from build123d import *

# Parameters (mm, degrees)
BOSS_EXTRUDE2_DEPTH = 15
SKETCH3_3_R         = 7.5
BOSS_EXTRUDE3_DEPTH = 20


with BuildPart() as part:
    # Sketch3 → Boss-Extrude2 (new body, symmetric)
    with BuildSketch(Plane.XY):
        Polygon((0, 0), (30, -30), (35, -30), (5, 0), align=None)
    extrude(amount=BOSS_EXTRUDE2_DEPTH, both=True)

    # Sketch3<3> → Boss-Extrude3 (add, symmetric)
    with BuildSketch(Plane.XY):
        with Locations((0.5, 6)):
            Circle(SKETCH3_3_R)
    extrude(amount=BOSS_EXTRUDE3_DEPTH, both=True)


solid = part.part
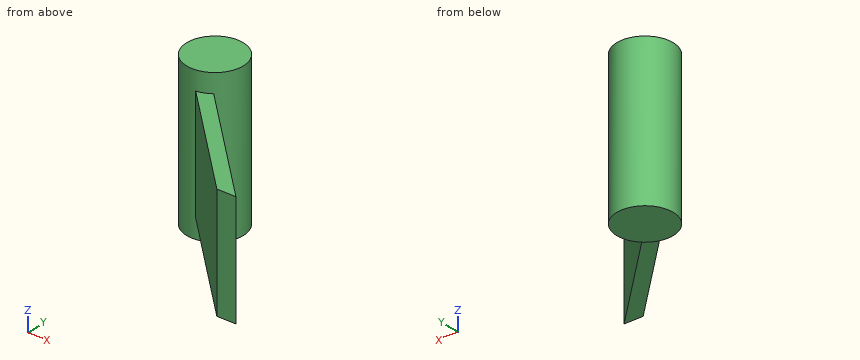
Geometry: final body of the model. Coordinates: model frame, mm. Give positions to 0.01 mm unless a question says otherwise; leave off trailing zeros. Loops run counter-clockwise (first coordinate to the right, second up) from the corner with the lowest first, then second, coordinate; pieces in that order, holes last. Notation, with made-up numbers: M -10.5,37 L 19.5,37 A31 ccw 19.5,65 Z; hole C 70,39.25 d2. An arc over 180 degrees is marked long. Put each result on its own line as item: value. Start each with the question number.
1) Cut plane A-A (x = 0.5). Output: boundary loops of the cut face in (y, z), then the cut area to 3 significant figures.
2) Cut plane B-B (y = 6). Output: boundary loops of the cut face in (x, z).
3) Ray query, line 1 along Y through (x, z) = (20, -9.5); line 2 along Y through (x, z) = (7, 11); line 3 along X through (y, z) = (-24.5, 4). Return the intervals inside material, ascending.
4) Contact query for flat-ended pins moving along their axis: pin 1 (9 mm diameter, centred on x = 24, y = -19, fed in from -Z); pin 2 (6 mm diameter, centred on y = -25.5, z = -12, fed in from -X); pin 3 (5 mm diameter, centred on y = -5.5, z = -2.5, fed in from -X). Output: stop coordinate, or through.
Verdict:
1. outline: M -1.5,-20 L 13.5,-20 L 13.5,20 L -1.5,20 Z
1. area: 600 mm2
2. outline: M -7,-20 L 8,-20 L 8,20 L -7,20 Z
3. line 1: -20 to -15
3. line 2: -7 to -2, 2.26 to 9.74
3. line 3: 24.5 to 29.5
4. pin 1: z = -15
4. pin 2: x = 22.5
4. pin 3: x = 3
